Geometry: final body of the model. Coordinates: model frame, mm. A direction names the side the tool comes from. Give positions to 0.01 mm unless a question says otherwise; leave off trailing zeros. Loops run counter-clockwise (first coordinate to the right, second up) from the corner with the lowest first, then second, coordinate; pieces in that order, holes last. Notation, with made-up numbers: (-24.5, 61.5) -> (30.5, 61.5) arc R16 ccw to (30.5, 65.5) -> close; hole circle Ø4 at (32, 6.5). An arc over 180 degrees is marked (long way). Answer in a Markdown table with one row per item. Add a question column.
1) Section query A-A (x = 8.75). Return the cut outline in (y, z), plus the area to 3 significant figures.
2) Section query C-C (x = 5). Return the cut outline in (y, z), plus the area to 3 significant figures.
3) First-contact query: P1, Ø0.9, axis at x = 6, z = 1.5, coming from the -Y side; P2, Ø1.5, axis at x = -9.5, z = 1, coming from the +Y side; P3, Ø0.6, axis at x = 6.5, z = 2, coming from the +Y side; P4, Ø5, axis at x = -7.5, y = -21.5, coming from the +Z side. Flat tips, straight axial feed; report the tip coordinate or a pass-through.
4) Draft query along Y for faces 1 (the flat face through (-7.155, -21.129, 1.232)), 2 (the cylindrical face through (8.623, -15.096, 1.232)), 3 (the flat face through (1, -15, 0)), 4 (the cylindrical face through (-13.52, -14.13, 1.23)). Return one class per face: +Y half, -Y half, draft (parallel to the pull), parting line (faces both ways), or undercut.
5) Section query D-D (y = -8.5). Give the number of separate pieces and of enclosed holes in the cut face, plus the area to 3 significant figures.
6) Section query B-B (y = -19.25). Return the cut outline in (x, z), plus the area to 3 significant figures.
7) Access query for faces 5 (the cylindrical face through (-0.016, -27.663, 1.232)), 6 (the flat face through (-0.624, -10, 1)). Directions: +Z, -Z, +X, -X, +Y, -Y. A direction counts if a zero-diameter tool reaches every point of the face in a straight line with its end or side. Return the directions, or none.
8) Line query: line 1 (X direction, y = -7.75, z = 2.3); line 2 (Y direction, x = -6, z = 0.55); line 3 (Y direction, x = 2, z = 1.5). Output: solid intervals per line, ascending. Write a range as from..to.
```python
from build123d import *

# Parameters (mm, degrees)
F1_DEPTH = 2.5
F2_R     = 0.85
F3_DEPTH = 12.5


with BuildPart() as f1:
    # F0 (on Top) → F1 (new body)
    with BuildSketch(Plane.XY):
        with BuildLine():
            Line((13.081475452, -13.081475452), (1.0606601718, -1.0606601718))
            ThreePointArc((1.0606601718, -1.0606601718), (0, -0.6213203436), (-1.0606601718, -1.0606601718))
            Line((-1.0606601718, -1.0606601718), (-13.081475452, -13.081475452))
            ThreePointArc((-13.081475452, -13.081475452), (-13.5208152802, -14.1421356237), (-13.081475452, -15.2027957955))
            Line((-13.081475452, -15.2027957955), (-1.0606601718, -27.2236110757))
            ThreePointArc((-1.0606601718, -27.2236110757), (0, -27.6629509039), (1.0606601718, -27.2236110757))
            Line((1.0606601718, -27.2236110757), (13.081475452, -15.2027957955))
            ThreePointArc((13.081475452, -15.2027957955), (13.5208152802, -14.1421356237), (13.081475452, -13.081475452))
        make_face()
        with BuildLine():
            add(Edge.make_bspline(
                [(-5.0351947703, -7.1148621023), (-3.1127377117, -7.1148621023), (-3.1127377117, -8.6094826309)],
                knots=[0, 0, 0, 1, 1, 1], degree=2))
            add(Edge.make_bspline(
                [(-3.1127377117, -8.6094826309), (-3.1127377117, -9.3887964152), (-3.6444453152, -9.8082109662)],
                knots=[0, 0, 0, 1, 1, 1], degree=2))
            add(Edge.make_bspline(
                [(-3.6444453152, -9.8082109662), (-4.1761529188, -10.2276255173), (-5.1654547112, -10.2276255173)],
                knots=[0, 0, 0, 1, 1, 1], degree=2))
            Line((-5.1654547112, -10.2276255173), (-5.7695913335, -10.2276255173))
            Line((-5.7695913335, -10.2276255173), (-5.7695913335, -12.2455316704))
            Line((-5.7695913335, -12.2455316704), (-6.3658674423, -12.2455316704))
            Line((-6.3658674423, -12.2455316704), (-6.3658674423, -7.1148621023))
            Line((-6.3658674423, -7.1148621023), (-5.0351947703, -7.1148621023))
        make_face(mode=Mode.SUBTRACT)
        with BuildLine():
            Line((-8.1334756687, -14.8039748892), (-8.1334756687, -13.4802963582))
            Line((-8.1334756687, -13.4802963582), (-0.6236797201, -13.4802963582))
            Line((-0.6236797201, -13.4802963582), (-0.6236797201, -6.9198086858))
            ThreePointArc((-0.6236797201, -6.9198086858), (-0.9032194318, -6.4583786209), (-0.9135835525, -5.9189782686))
            ThreePointArc((-0.9135835525, -5.9189782686), (0.0168397474, -5.0141534426), (0.9868078824, -5.876451129))
            ThreePointArc((0.9868078824, -5.876451129), (0.9900106564, -6.4384308628), (0.6999988109, -6.9198086858))
            Line((0.6999988109, -6.9198086858), (0.6999988109, -13.4802963582))
            Line((0.6999988109, -13.4802963582), (8.1334756687, -13.4802963582))
            ThreePointArc((8.1334756687, -13.4802963582), (8.5949057336, -13.2007566465), (9.134306086, -13.1903925258))
            ThreePointArc((9.134306086, -13.1903925258), (10.0391309119, -14.1208158258), (9.1768332255, -15.0907839607))
            ThreePointArc((9.1768332255, -15.0907839607), (8.6148534917, -15.0939867347), (8.1334756687, -14.8039748892))
            Line((8.1334756687, -14.8039748892), (0.6999988109, -14.8039748892))
            Line((0.6999988109, -14.8039748892), (0.6999988109, -23.1867600232))
            Line((0.6999988109, -23.1867600232), (-0.6236797201, -23.1867600232))
            Line((-0.6236797201, -23.1867600232), (-0.6236797201, -14.8039748892))
            Line((-0.6236797201, -14.8039748892), (-8.1334756687, -14.8039748892))
        make_face(mode=Mode.SUBTRACT)
        with BuildLine():
            Line((4.4893827087, -12.0222926794), (4.0456231809, -12.0222926794))
            Line((4.0456231809, -12.0222926794), (2.4385501247, -7.8231663068))
            Line((2.4385501247, -7.8231663068), (2.4126295915, -7.8231663068))
            add(Edge.make_bspline(
                [(2.4126295915, -7.8231663068), (2.4582497299, -8.3218773648), (2.4582497299, -9.0092899044)],
                knots=[0, 0, 0, 1, 1, 1], degree=2))
            Line((2.4582497299, -9.0092899044), (2.4582497299, -12.0222926794))
            Line((2.4582497299, -12.0222926794), (1.9491704586, -12.0222926794))
            Line((1.9491704586, -12.0222926794), (1.9491704586, -7.2850560383))
            Line((1.9491704586, -7.2850560383), (2.7786275198, -7.2850560383))
            Line((2.7786275198, -7.2850560383), (4.2789079794, -11.1928356181))
            Line((4.2789079794, -11.1928356181), (4.3048285126, -11.1928356181))
            Line((4.3048285126, -11.1928356181), (5.817550828, -7.2850560383))
            Line((5.817550828, -7.2850560383), (6.6407869613, -7.2850560383))
            Line((6.6407869613, -7.2850560383), (6.6407869613, -12.0222926794))
            Line((6.6407869613, -12.0222926794), (6.0902348369, -12.0222926794))
            Line((6.0902348369, -12.0222926794), (6.0902348369, -8.969890694))
            add(Edge.make_bspline(
                [(6.0902348369, -8.969890694), (6.0902348369, -8.4452591027), (6.1358549753, -7.8293872347)],
                knots=[0, 0, 0, 1, 1, 1], degree=2))
            Line((6.1358549753, -7.8293872347), (6.1099344421, -7.8293872347))
            Line((6.1099344421, -7.8293872347), (4.4893827087, -12.0222926794))
        make_face(mode=Mode.SUBTRACT)
    extrude(amount=F1_DEPTH)

    # F2 (on Right) → F3 (cut, symmetric)
    with BuildSketch(Plane.YZ):
        with Locations((-2.4908210296, 1.292226194)):
            Circle(F2_R)
    extrude(amount=F3_DEPTH, both=True, mode=Mode.SUBTRACT)


solid = f1.part
```
Evaluation:
| question | item | result |
|---|---|---|
| 1 | outline | (-19.53, 0) -> (-15.12, 0) -> (-15.12, 2.5) -> (-19.53, 2.5) -> close; (-13.17, 0) -> (-8.75, 0) -> (-8.75, 2.5) -> (-13.17, 2.5) -> close |
| 1 | area | 22.1 mm² |
| 2 | outline | (-23.28, 0) -> (-14.8, 0) -> (-14.8, 2.5) -> (-23.28, 2.5) -> close; (-13.48, 0) -> (-10.7, 0) -> (-10.7, 2.5) -> (-13.48, 2.5) -> close; (-9.4, 0) -> (-5, 0) -> (-5, 2.5) -> (-9.4, 2.5) -> close |
| 2 | area | 39.1 mm² |
| 3 | P1 | y = -22.73 |
| 3 | P2 | y = -8.75 |
| 3 | P3 | y = -6.2 |
| 3 | P4 | z = 2.5 |
| 4 | face 1 | -Y half |
| 4 | face 2 | undercut |
| 4 | face 3 | draft |
| 4 | face 4 | parting line |
| 5 | separate pieces | 7 |
| 5 | enclosed holes | 0 |
| 5 | area | 25.8 mm² |
| 6 | outline | (-9.03, 0) -> (-0.62, 0) -> (-0.62, 2.5) -> (-9.03, 2.5) -> close; (0.7, 0) -> (9.03, 0) -> (9.03, 2.5) -> (0.7, 2.5) -> close |
| 6 | area | 41.9 mm² |
| 7 | face 5 | +Z, -Z, -Y |
| 7 | face 6 | +Z, -Z |
| 8 | line 1 | -7.75..-6.37, -3.35..-0.62, 0.7..1.95, 2.96..5.64, 6.64..7.75 |
| 8 | line 2 | -22.28..-14.8, -13.48..-12.25, -7.11..-6 |
| 8 | line 3 | -26.28..-14.8, -13.48..-12.02, -7.29..-3.32 |
